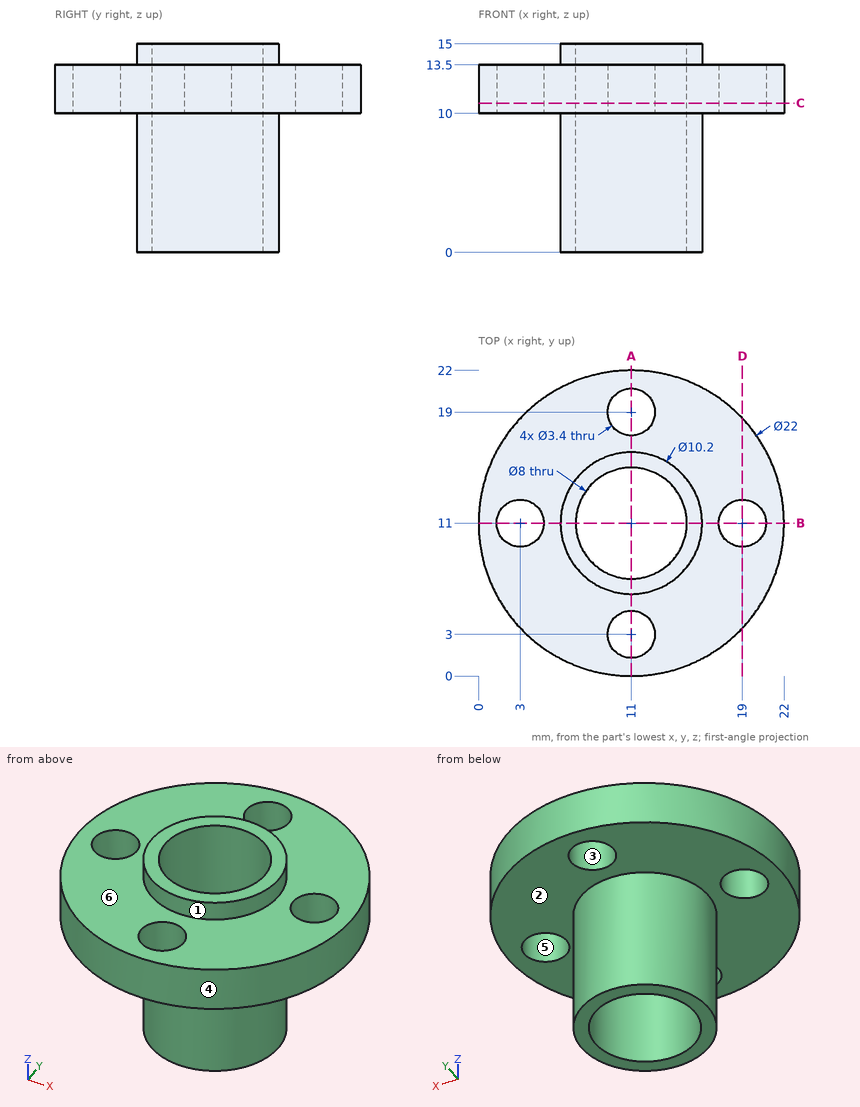
Answer from the drawing. Dimensions are ordinates in mm from the lowest x, y and z of the part. A direction names the side the tool comes from. Give positions to 0.01 mm unless a question says otherwise; leave off trailing zeros. Loops run counter-clockwise (first coordinate to the right, second up) from the corner with the lowest first, then second, coordinate; pieces in that order, holes last.
Item 1: Find the intervals of material crossed by line 1 along X through (y, z) = (11, 12.5); line 2 along Y through (x, z) = (11, 4.5), in increasing order.
Item 2: The part is cut by section C-C (z = 10.75). Write down the section's boundary in (x, y).
Item 3: The part is cut by section D-D (x = 19). Write down the section's boundary in (y, z), and give its area (3 significant figures).
Item 4: Each of these flat-tipped pins is pushed along its axis until it touches: pin 1 Ø4.5 at (x, y) = (11, 3) entering from +Z; pin 2 Ø6 at (y, z) = (17, 6.5) entering from +X; pin 3 Ø1.5 at (y, z) = (7, 9) entering from -X. Where does it stop, or does it pass through?
Item 5: For the marked faces 1, 2 and 3, determine the directions among +Z, -Z, +X, -X, +Y, -Y from which every point of the face is accessible in a straight line to the end or side of a thin tool.
Item 6: The part is cut by section A-A (x = 11). Write down the section's boundary in (y, z), and give its area (3 significant figures).
Item 7: The mould has two halves that part along Y. Classify the marked faces 4, 5 and 6: released by +Y, released by -Y, zero draft, split by the parting line, or undercut.
Taken from the geometry:
1. line 1: x = 0 to 1.3, 4.7 to 7, 15 to 17.3, 20.7 to 22
1. line 2: y = 5.9 to 7, 15 to 16.1
2. outline: circle Ø22 at (11, 11); hole circle Ø3.4 at (3, 11); hole circle Ø8 at (11, 11); hole circle Ø3.4 at (11, 3); hole circle Ø3.4 at (11, 19); hole circle Ø3.4 at (19, 11)
3. outline: (3.45, 10) - (9.3, 10) - (9.3, 13.5) - (3.45, 13.5) - close; (12.7, 10) - (18.55, 10) - (18.55, 13.5) - (12.7, 13.5) - close
3. area: 40.9 mm2
4. pin 1: stops at z = 13.5
4. pin 2: stops at x = 15.12
4. pin 3: stops at x = 7.07
5. face 1: +Z
5. face 2: -Z
5. face 3: +Z, -Z
6. outline: (0, 10) - (1.3, 10) - (1.3, 13.5) - (0, 13.5) - close; (4.7, 10) - (5.9, 10) - (5.9, 0) - (7, 0) - (7, 15) - (5.9, 15) - (5.9, 13.5) - (4.7, 13.5) - close; (15, 0) - (16.1, 0) - (16.1, 10) - (17.3, 10) - (17.3, 13.5) - (16.1, 13.5) - (16.1, 15) - (15, 15) - close; (20.7, 10) - (22, 10) - (22, 13.5) - (20.7, 13.5) - close
6. area: 50.5 mm2
7. face 4: split by the parting line
7. face 5: undercut
7. face 6: zero draft
